Check sheet for the modelled part. Datum: model origin and axes. Units: mm. A direction names the side the tool comes from. Round coordinates to 2 decimals unless told otherwise and drop trailing zeros. Answer in a Markdown table with one row per item.
```python
from build123d import *


with BuildPart() as part:
    # Sketch1 → Revolve1 (revolve)
    with BuildSketch(Plane(origin=(0, 0, 0), x_dir=(0, 0, -1), z_dir=(1, 0, 0)), mode=Mode.PRIVATE) as revolve1_sk:
        with BuildLine():
            Line((0, 41.25), (0, 49.675))
            ThreePointArc((0, 49.675), (0.146446609, 50.028553391), (0.5, 50.175))
            Line((0.5, 50.175), (4.478693294, 50.175))
            ThreePointArc((4.478693294, 50.175), (4.999293087, 50.188560401), (5.518480971, 50.229204829))
            Line((5.518480971, 50.229204829), (10.5, 50.75))
            Line((10.5, 50.75), (12, 49.25))
            Line((12, 49.25), (12, 47.5))
            Line((12, 47.5), (7.711429508, 46.207458652))
            ThreePointArc((7.711429508, 46.207458652), (7.000073654, 45.237863155), (7.734753866, 44.285819266))
            Line((7.734753866, 44.285819266), (11.5, 43.25))
            Line((11.5, 43.25), (11.5, 41))
            Line((11.5, 41), (10.633974596, 39.5))
            Line((10.633974596, 39.5), (7.915505944, 40.321990009))
            ThreePointArc((7.915505944, 40.321990009), (6.484090894, 40.642418817), (5.021199936, 40.75))
            Line((5.021199936, 40.75), (0.5, 40.75))
            ThreePointArc((0.5, 40.75), (0.146446609, 40.896446609), (0, 41.25))
        make_face()
    revolve(revolve1_sk.sketch.rotate(Axis((0, 0, 0), (0, 0, -1)), 90), axis=Axis((0, 0, 0), (0, 0, -1)))


solid = part.part
```
(1) Tool access check on faces 1 (the cylindrical face through (37.64, 15.61, -2.73)), 2 (the flat face through (-7, -41, 0)), 3 (the flat face through (16, 38, -11.5)). Record the directions out of +Z, -Z, +X, -X, +Y, -Y that give a thin tool (end or side, any length) a straight path to the whole face; none if there is none.
Solutions:
| item | result |
|---|---|
| face 1 | +Z |
| face 2 | +Z, +X, -X, +Y, -Y |
| face 3 | -Z |
(2) Draft check along Y on faces 4 (the cylindrical face through (47.86, -15.07, -2.52)), 5 (the flat face through (-26, -40, -12)), 6 (the conical face through (-9.39, 42.27, -11.32)). Enter one of: pulls with the +Y half, pulls with the -Y half, needs draft (parallel to the pull), parting line crosses it, or undercut.
Solutions:
| item | result |
|---|---|
| face 4 | parting line crosses it |
| face 5 | needs draft |
| face 6 | undercut |
(3) Depth check by flat-ended pin: pin 1 Ø4 at (y, z) = (11.5, -5.5) entering from +X; pin 2 Ø1.5 at (y, z) = (34, -5) entering from +X; pin 3 Ø6 at (y, z) = (4.5, -9.5) entering from +X. Enter the tip coordinate at first touch or a pass-through.
Solutions:
| item | result |
|---|---|
| pin 1 | x = 49.38 |
| pin 2 | x = 37.6 |
| pin 3 | x = 50.72 |
(4) Scan lines: probe 1 along X at (y, z) = (23, -7.5); probe 2 along Y at (x, z) = (-22, -10.25); probe 3 along Y at (x, z) = (-28, -10.5). Record each from-to range of solid material in increasing order. Write a range as from..to.
Solutions:
| item | result |
|---|---|
| probe 1 | -44.89..-39.97, -37.96..-33.26, 33.26..37.96, 39.97..44.89 |
| probe 2 | -45.7..-41.5, -37.64..-32.95, 32.95..37.64, 41.5..45.7 |
| probe 3 | -42.33..-37.81, -33.32..-27.92, 27.92..33.32, 37.81..42.33 |
